Read the model definition and answer for the solid it produces. Units are mm, in the model's axes. Face numbers are marked on the shaded views. A direction names the side the tool comes from. Coordinates: 2 decimals unless noted, no trailing zeros.
1) Find the intervals of material crossed by line 1 (Y direction, x = -2.5, z = 3.75); line 2 (Y direction, x = 3, z = 0); line 3 (X direction, y = 31, z = 2.5), in increasing order.
2) Determine the mould class of the marked faces 1, 2 and 3 for opening direction Z: +Z half, -Z half, draft (parallel to the pull), parting line (faces both ways), or undercut.
3) Which of the six approach directions +Z, -Z, +X, -X, +Y, -Y give full straight-line access (tool end or side, diameter ignored) to the marked faces 4, 5 and 6?
4) Each of these flat-tipped pins is pushed along its axis until it touches: pin 1 Ø3 at (x, z) = (-0.5, 0.5) entering from +Y; pin 2 Ø2 at (x, y) = (2.5, 14) entering from +Z; pin 3 Ø1.5 at (y, z) = (16, 0) entering from +X. Where does it stop, or does it pass through?
from build123d import *

# Parameters (mm, degrees)
CUT_EXTRUDE_1_DEPTH = 4


with BuildPart() as part:
    # 草图1 → 旋转1 (revolve)
    with BuildSketch(Plane.XY, mode=Mode.PRIVATE) as revolve_1_sk:
        with BuildLine():
            Line((0, 0), (0, 32.8))
            Line((0, 32.8), (4.65, 32.8))
            ThreePointArc((4.65, 32.8), (5.357106781, 32.507106781), (5.65, 31.8))
            Line((5.65, 31.8), (5.65, 25))
            Line((5.65, 25), (4, 25))
            Line((4, 25), (3.4, 24.577341211))
            Line((3.4, 24.577341211), (4, 24.154682421))
            Line((4, 24.154682421), (3.4, 23.732023632))
            Line((3.4, 23.732023632), (4, 23.309364843))
            Line((4, 23.309364843), (3.4, 22.886706054))
            Line((3.4, 22.886706054), (4, 22.464047264))
            Line((4, 22.464047264), (3.4, 22.041388475))
            Line((3.4, 22.041388475), (4, 21.618729686))
            Line((4, 21.618729686), (3.4, 21.196070897))
            Line((3.4, 21.196070897), (4, 20.773412107))
            Line((4, 20.773412107), (3.4, 20.350753318))
            Line((3.4, 20.350753318), (4, 19.928094529))
            Line((4, 19.928094529), (3.4, 19.50543574))
            Line((3.4, 19.50543574), (4, 19.08277695))
            Line((4, 19.08277695), (3.4, 18.660118161))
            Line((3.4, 18.660118161), (4, 18.237459372))
            Line((4, 18.237459372), (3.4, 17.814800583))
            Line((3.4, 17.814800583), (4, 17.392141793))
            Line((4, 17.392141793), (3.4, 16.969483004))
            Line((3.4, 16.969483004), (4, 16.546824215))
            Line((4, 16.546824215), (3.4, 16.124165426))
            Line((3.4, 16.124165426), (4, 15.701506636))
            Line((4, 15.701506636), (3.4, 15.278847847))
            Line((3.4, 15.278847847), (4, 14.856189058))
            Line((4, 14.856189058), (3.4, 14.433530269))
            Line((3.4, 14.433530269), (4, 14.010871479))
            Line((4, 14.010871479), (3.4, 13.58821269))
            Line((3.4, 13.58821269), (4, 13.165553901))
            Line((4, 13.165553901), (3.4, 12.742895112))
            Line((3.4, 12.742895112), (4, 12.320236322))
            Line((4, 12.320236322), (3.4, 11.897577533))
            Line((3.4, 11.897577533), (4, 11.474918744))
            Line((4, 11.474918744), (3.4, 11.052259955))
            Line((3.4, 11.052259955), (4, 10.629601165))
            Line((4, 10.629601165), (3.4, 10.206942376))
            Line((3.4, 10.206942376), (4, 9.784283587))
            Line((4, 9.784283587), (3.4, 9.361624798))
            Line((3.4, 9.361624798), (4, 8.938966008))
            Line((4, 8.938966008), (3.4, 8.516307219))
            Line((3.4, 8.516307219), (4, 8.09364843))
            Line((4, 8.09364843), (3.4, 7.67098964))
            Line((3.4, 7.67098964), (4, 7.248330851))
            Line((4, 7.248330851), (3.4, 6.825672062))
            Line((3.4, 6.825672062), (4, 6.403013273))
            Line((4, 6.403013273), (3.4, 5.980354483))
            Line((3.4, 5.980354483), (4, 5.557695694))
            Line((4, 5.557695694), (3.4, 5.135036905))
            Line((3.4, 5.135036905), (4, 4.712378116))
            Line((4, 4.712378116), (3.4, 4.289719326))
            Line((3.4, 4.289719326), (4, 3.867060537))
            Line((4, 3.867060537), (3.4, 3.444401748))
            Line((3.4, 3.444401748), (4, 3.021742959))
            Line((4, 3.021742959), (3.4, 2.599084169))
            Line((3.4, 2.599084169), (4, 2.17642538))
            Line((4, 2.17642538), (3.4, 1.753766591))
            Line((3.4, 1.753766591), (4, 1.331107802))
            Line((4, 1.331107802), (3.4, 0.908449012))
            Line((3.4, 0.908449012), (3.991663039, 0.491663039))
            Line((3.991663039, 0.491663039), (3.5, 0))
            Line((3.5, 0), (0, 0))
        make_face()
    revolve(revolve_1_sk.sketch.rotate(Axis((0, 31.8, 0), (0, 1, 0)), 90), axis=Axis((0, 31.8, 0), (0, 1, 0)))

    # 草图3 → 切除-拉伸1 (cut)
    with BuildSketch(Plane(origin=(0, 32.8, 0), x_dir=(1, 0, 0), z_dir=(0, 1, 0))):
        Polygon((3.464101615, 0), (1.732050808, 3), (-1.732050808, 3), (-3.464101615, 0), (-1.732050808, -3), (1.732050808, -3), align=None)
    extrude(amount=-CUT_EXTRUDE_1_DEPTH, mode=Mode.SUBTRACT)


solid = part.part
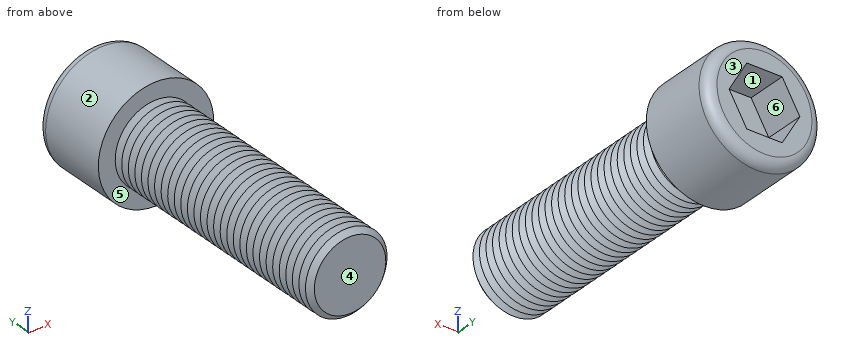
Reported:
1. line 1: y = 25 to 32.8
1. line 2: y = 0 to 28.8
1. line 3: x = -5.07 to -2.02, 2.02 to 5.07
2. face 1: undercut
2. face 2: parting line
2. face 3: draft
3. face 4: +Z, -Z, +X, -X, -Y
3. face 5: -Y
3. face 6: +Y
4. pin 1: stops at y = 28.8
4. pin 2: stops at z = 3.71
4. pin 3: stops at x = 4
